Autodesk Inventor part; units mm, degrees
ref_plane "YZ Plane" through (0, 0, 0) normal (1, 0, 0) x (0, 1, 0)
ref_plane "XZ Plane" through (0, 0, 0) normal (0, 1, 0) x (-1, 0, 0)
ref_plane "XY Plane" through (0, 0, 0) normal (0, 0, 1) x (1, 0, 0)
sketch "Boceto1" plane through (0, 0, 0) normal (0, 1, 0) x (-1, 0, 0)
  line L0 (15, 15) -> (-15, 15)
  line L1 (-15, 15) -> (-15, -15)
  line L2 (-15, -15) -> (15, -15)
  line L3 (15, -15) -> (15, 15)
  line L4 (15, 15) -> (-15, -15) construction
  circle A0 centre (0, 0) radius 4
  dimension "d0" = 30
  dimension "d1" = 8
extrude "Extrusión1" add sketch "Boceto1" along normal blind 426.5
properties part number "P_3030_1500"
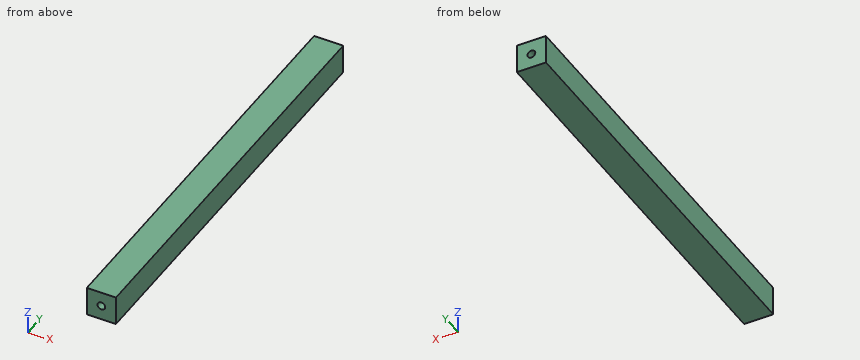
Check sheet for the modelled part. Datum: model origin and axes. Units: mm. Coordinates: 2 decimals unless noted, no trailing zeros. Write each loop counter-clockwise with the first axis right and the second up, starting at its lowest first coordinate (ties: lowest second). Pieces come first, ordered by that corner, then holes. Notation, with made-up numbers: M 78.25,79 L 84.25,79 A37 cw 84.25,116 Z; hole C 0.25,-23 d9. An arc over 180 degrees is marked long. Answer as CSV lines item,"result".
Q1. Material ranges on probe 1 along Z at (x, y) = (0, 191); probe 2 along X at (y, z) = (321, -0.5); probe 3 along X at (y, z) = (40.5, -3.25), recorded low to high. Write a range as from..to.
Check result:
probe 1,"-15..-4, 4..15"
probe 2,"-15..-3.97, 3.97..15"
probe 3,"-15..-2.33, 2.33..15"
Q2. Go/stop test with a flat-tipped pin: pin 1 (7 mm diameter, centred on x = 0, z = 0, fed in from -Y). Record where the tip stops, or that it passes through.
Check result:
pin 1,"through"
Q3. Cross-section at A-A (x = 0). Record the boundary of the cut face in (y, z).
Check result:
outline,"M 0,-15 L 426.5,-15 L 426.5,-4 L 0,-4 Z; M 0,4 L 426.5,4 L 426.5,15 L 0,15 Z"
Q4. Cross-section at C-C (y = 217.5). Record the boundary of the cut face in (x, z), then the cut area to 3 significant figures.
Check result:
outline,"M -15,-15 L 15,-15 L 15,15 L -15,15 Z; hole C 0,0 d8"
area,"850 mm^2"
Q5. Cross-section at B-B (z = 0). Record the boundary of the cut face in (x, y).
Check result:
outline,"M -15,0 L -4,0 L -4,426.5 L -15,426.5 Z; M 4,0 L 15,0 L 15,426.5 L 4,426.5 Z"
